Part print with two shaded views. Sizes in mm from the minimum x, y, z corner. Give positions to 0.01 mm unless a question says otherwise; leave off trailing zeros. Loops run counter-clockwise (first coordinate to the right, second up) from the corner with the lowest first, then second, coordinate; pieces in that order, holes last. Notation, with made-up numbers: (-7.75, 32.5) -> (2.25, 32.5) arc R21 ccw to (2.25, 70.5) -> close; hole circle Ø11 at (23, 54.25). An arc over 180 degrees is marked (long way). One line per question, with ' | ' between items. Start each with the question number.
(1) Flat gauge pins, fed straight in: pin 1 Ø3.5 at (x, y) = (3, 33) entering from -Z; pin 2 Ø2 at (y, z) = (8, 2) entering from +X; pin 3 Ø5 at (x, y) = (3, 3) entering from +Z; pin 4 Ø1 at (y, z) = (25, 2) entering from +X. Where does each tip first touch, or does it go through?
(2) Slice it at B-B, the plane x = 3. Write the cut outline in (y, z) (1 decimal).
(3) Mould opens along Y. For the marked faces 1 and 2 say: pulls with the +Y half, pulls with the -Y half, needs draft (parallel to the pull), parting line crosses it, or undercut.
(4) Slice it at A-A, the plane z = 1.45. Give the number of separate pieces and of enclosed holes in the cut face.
(5) Slice it at D-D, the plane x = 8. Write the cut outline in (y, z) (1 decimal).
(6) Drill centre lines: L1, parallel to Y at x = 3, z = 1.25 (1 decimal); L2, parallel to X at y = 4.5, z = 1.75 (1 decimal). Where is each one in solid material? Low to high. Write a range as from..to.
(7) Slice it at C-C, the plane y = 3.5. Write the cut outline in (x, z).
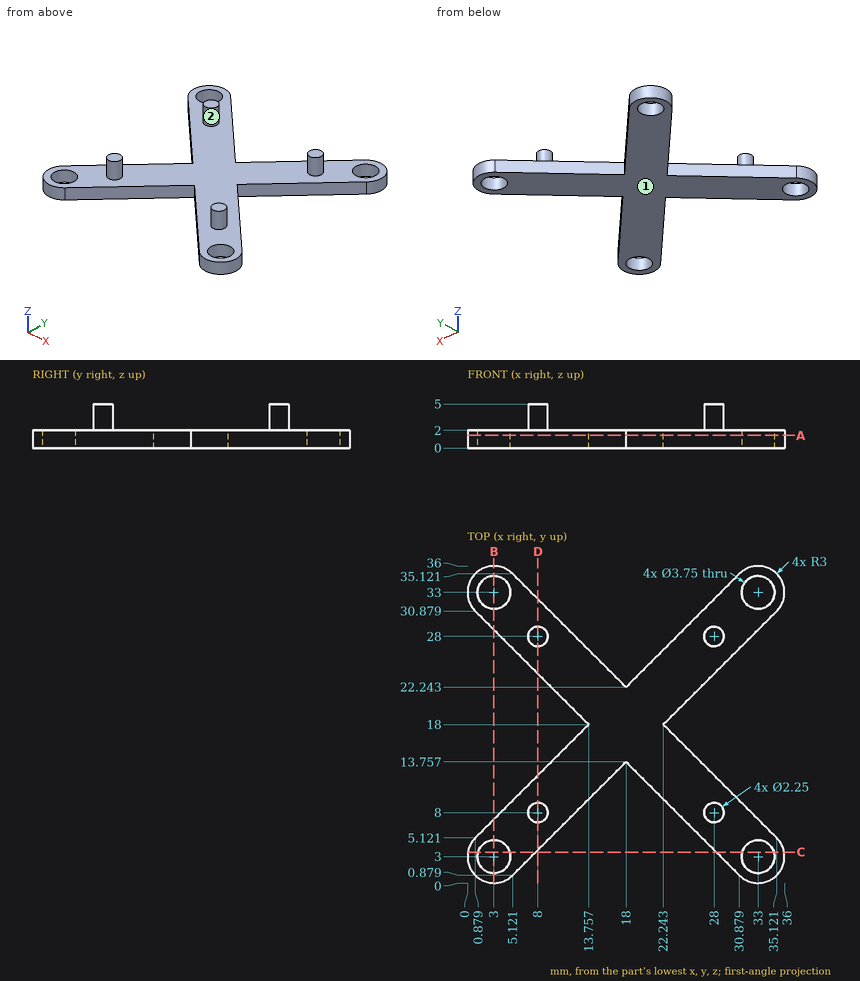
Final values:
1) pin 1: through | pin 2: x = 33.24 | pin 3: z = 2 | pin 4: x = 29.74
2) outline: (0, 0) -> (1.1, 0) -> (1.1, 2) -> (0, 2) -> close; (4.9, 0) -> (7.2, 0) -> (7.2, 2) -> (4.9, 2) -> close; (28.8, 0) -> (31.1, 0) -> (31.1, 2) -> (28.8, 2) -> close; (34.9, 0) -> (36, 0) -> (36, 2) -> (34.9, 2) -> close
3) face 1: needs draft | face 2: undercut
4) separate pieces: 1 | enclosed holes: 4
5) outline: (3.8, 0) -> (12.2, 0) -> (12.2, 2) -> (9.1, 2) -> (9.1, 5) -> (6.9, 5) -> (6.9, 2) -> (3.8, 2) -> close; (23.8, 0) -> (32.2, 0) -> (32.2, 2) -> (29.1, 2) -> (29.1, 5) -> (26.9, 5) -> (26.9, 2) -> (23.8, 2) -> close
6) L1: 0..1.1, 4.9..7.2, 28.8..31.1, 34.9..36 | L2: 0.4..1.9, 4.1..8.7, 27.3..31.9, 34.1..35.6
7) outline: (0.04, 0) -> (1.19, 0) -> (1.19, 2) -> (0.04, 2) -> close; (4.81, 0) -> (7.74, 0) -> (7.74, 2) -> (4.81, 2) -> close; (28.26, 0) -> (31.19, 0) -> (31.19, 2) -> (28.26, 2) -> close; (34.81, 0) -> (35.96, 0) -> (35.96, 2) -> (34.81, 2) -> close
